from build123d import *

# Parameters (mm, degrees)
BOSS_EXTRUDE1_DEPTH     = 20
FILLET1_R               = 4
SKETCH2_R               = 2.75
CUT_EXTRUDE1_DEPTH      = 1.5
LPATTERN1_COUNT         = 2
LPATTERN1_PITCH         = 30
CUT_EXTRUDE2_DEPTH      = 35.641016151
CUT_EXTRUDE2_DEPTH_BACK = 35.641016151
WRAP1_DEPTH             = 1


# Read off the part's stored shape, not the designer's step: Wrap1
with BuildPart() as part:
    # Sketch1 → Boss-Extrude1 (new body)
    with BuildSketch(Plane(origin=(0, 0, 0), x_dir=(1, 0, 0), z_dir=(0, 1, 0))):
        with BuildLine():
            Line((-15, -5), (10, -5))
            Line((10, -5), (10, -15))
            ThreePointArc((10, -15), (15, -20), (20, -15))
            Line((20, -15), (20, 0))
            ThreePointArc((20, 0), (18.535533906, 3.535533906), (15, 5))
            Line((15, 5), (-15, 5))
            ThreePointArc((-15, 5), (-20, 0), (-15, -5))
        make_face()
    extrude(amount=BOSS_EXTRUDE1_DEPTH)

    # Fillet1
    fillet1_edges = [part.edges().sort_by_distance(p)[0] for p in [
        (15, 20, 20),
        (20, 20, 7.5),
        (18.535533906, 20, -3.535533906),
        (0, 20, -5),
        (-20, 20, 0),
        (-2.5, 20, 5),
        (10, 20, 10),
    ]]
    fillet(fillet1_edges, radius=FILLET1_R)

    # Sketch2 → Cut-Extrude1 (cut)
    with BuildSketch(Plane.XZ):
        with Locations(Location((-15, 0, 0), (0, 0, 270))):
            Circle(SKETCH2_R)
    cut_extrude1 = extrude(amount=-CUT_EXTRUDE1_DEPTH, mode=Mode.SUBTRACT)

    # LPattern1: Cut-Extrude1 ×2
    with Locations(*[(i * LPATTERN1_PITCH, 0, 0) for i in range(1, LPATTERN1_COUNT)]):
        add(cut_extrude1, mode=Mode.SUBTRACT)

    # Sketch3 → Cut-Extrude2 (cut, two sides: drawn at the far end of the back side and taken through both)
    with BuildSketch(Plane.XY.offset(-CUT_EXTRUDE2_DEPTH_BACK)):
        with BuildLine():
            Line((5, 17), (-5, 17))
            ThreePointArc((-5, 17), (-8, 20), (-5, 23))
            Line((-5, 23), (5, 23))
            ThreePointArc((5, 23), (8, 20), (5, 17))
        make_face()
    extrude(amount=CUT_EXTRUDE2_DEPTH + CUT_EXTRUDE2_DEPTH_BACK, mode=Mode.SUBTRACT)

    # Wrap1 outline → Wrap1 (add)
    with BuildSketch(Plane(origin=(0, 17, 0), x_dir=(1, 0, 0), z_dir=(0, 1, 0))):
        with BuildLine():
            add(Edge.make_bspline(
                [(1.841863893, -2.738252863), (1.843167117, -2.772610038), (1.845627679, -2.837478309), (1.870220056, -2.928234816), (1.910417773, -3.005660397), (1.968656697, -3.069246584), (2.04558102, -3.11604167), (2.138808991, -3.149069173), (2.249599225, -3.170094309), (2.329470455, -3.171691186), (2.372312611, -3.172547735)],
                knots=[0, 0, 0, 0, 0.130861591, 0.247074017, 0.355594274, 0.460908048, 0.571758266, 0.695587752, 0.836716212, 1, 1, 1, 1], degree=3))
            Line((1.841863893, -2.738252863), (1.841863893, -1.839214402))
            Line((1.841863893, -1.839214402), (2.970069021, -1.839214402))
            Line((2.970069021, -1.839214402), (2.970069021, -1.223829786))
            Line((2.970069021, -1.223829786), (1.841863893, -1.223829786))
            Line((1.841863893, -1.223829786), (1.841863893, 4.006939444))
            Line((1.841863893, 4.006939444), (1.295389534, 4.006939444))
            Line((1.295389534, 4.006939444), (-2.465828415, -1.130881068))
            Line((-2.465828415, -1.130881068), (-2.465828415, -1.839214402))
            Line((-2.465828415, -1.839214402), (0.303402354, -1.839214402))
            Line((0.303402354, -1.839214402), (0.303402354, -2.579599017))
            add(Edge.make_bspline(
                [(0.154363893, -3.050752863), (0.177887379, -3.022926473), (0.227059219, -2.964760144), (0.27088721, -2.852439848), (0.29873926, -2.722573798), (0.301775942, -2.629466316), (0.303402354, -2.579599017)],
                knots=[0, 0, 0, 0, 0.214745145, 0.448888149, 0.704830817, 1, 1, 1, 1], degree=3))
            add(Edge.make_bspline(
                [(-0.279930979, -3.172547735), (-0.230645452, -3.171172689), (-0.140021776, -3.168644324), (-0.016795191, -3.146993527), (0.083806957, -3.111501143), (0.132261074, -3.069783001), (0.154363893, -3.050752863)],
                knots=[0, 0, 0, 0, 0.31964973, 0.587755386, 0.811950592, 1, 1, 1, 1], degree=3))
            Line((-0.279930979, -3.172547735), (-0.824802774, -3.172547735))
            Line((-0.824802774, -3.172547735), (-0.824802774, -3.685368248))
            Line((-0.824802774, -3.685368248), (2.662376713, -3.685368248))
            Line((2.662376713, -3.685368248), (2.662376713, -3.172547735))
            Line((2.662376713, -3.172547735), (2.372312611, -3.172547735))
        make_face()
        Polygon((0.303402354, 1.822644573), (0.303402354, -1.223829786), (-1.927366876, -1.223829786), align=None, mode=Mode.SUBTRACT)
    extrude(amount=WRAP1_DEPTH)


solid = part.part
Verification items for the finished model (mm, model axes). A direction names the side the tool comes from. Coordinates: 2 decimals unless noted, no trailing zeros. Order: outer loops, then holes, each group sorted by start corner. A loop starts at its lowest first (then second) coordinate and runs counter-clockwise, first axis right, second up. Notation, with made-up numbers: M 34.25,15 L 79.25,15 A24 cw 79.25,51 Z; hole C 30,-22 d5. An arc over 180 degrees is marked long. Return JSON: item names as keys, results as strings.
1) Gauge pin test, flat ends, axial feed: pin 1 (1 mm diameter, centred on x = -6.5, y = 14, fed in from +Z); pin 2 (0.6 mm diameter, centred on x = 1.5, y = 17.5, fed in from -Z); pin 3 (0.8 mm diameter, centred on x = 2.5, y = 17.5, fed in from +Z). Record the tip position at first contact, or that the pin passes through.
Answer list:
{"pin 1": "z = 5", "pin 2": "z = -4.01", "pin 3": "z = 3.69"}
2) Cross-section at C-C, the plane y = 5.75. Record the boundary of the cut face in (x, z).
Answer list:
{"outline": "M -15,-5 L 15,-5 A5 ccw 20,0 L 20,15 A5 ccw 10,15 L 10,5 L -15,5 A5 ccw Z"}
3) Cross-section at A-A, the plane z = 13. Record the boundary of the cut face in (x, y).
Answer list:
{"outline": "M 10,0 L 20,0 L 20,16 A4 ccw 16,20 L 14,20 A4 ccw 10,16 Z"}
4) Access from +Z, -Z, +X, -X, +Y, -Y to the whole of each face (thin tool, end or side, straight path). Record for faces 4 (the flat face through (2.4, 17.5, 1.224)), 5 (the flat face through (15, 1.5, 0)), 6 (the flat face through (1.842, 17.5, 2.3)), 7 (the cylindrical face through (-3.52, 16.3, 4.99)).
Answer list:
{"face 4": "-Z, +Y", "face 5": "-Y", "face 6": "+Y", "face 7": "+Z, -X, +Y"}
5) Release check for a two-part mould opening along X. For faces 1 (the flat face through (-12, 20, 0)), 2 (the flat face through (1, 18, 1)), 3 (the cylindrical face through (15, 8, 20)) record: +X half, -X half, draft (parallel to the pull), parting line (faces both ways), or undercut.
Answer list:
{"face 1": "draft", "face 2": "undercut", "face 3": "parting line"}
6) Thickness scan on L1, parallel to X at y = 0.3, z = 0; L2, parallel to Z at x = -1.5, y = 8; L3, parallel to X at y = 3.25, z = 13. Record the ranges inside material, lowest first. Write a range as [from, to].
Answer list:
{"L1": "[-20, -17.75], [-12.25, 12.25], [17.75, 20]", "L2": "[-5, 5]", "L3": "[10, 20]"}
7) Cross-section at B-B, the plane x = -10.5. Record the boundary of the cut face in (y, z), and give its area (3 significant figures).
Answer list:
{"outline": "M 0,-5 L 16,-5 A4 ccw 20,-1 L 20,1 A4 ccw 16,5 L 0,5 Z", "area": "193 mm2"}
